Geometry: final body of the model. Coordinates: model frame, mm. A direction names the side the tool comes from. Round coordinates to 2 decimals unless told otherwise and drop trailing zeros. Loops run counter-clockwise (first coordinate to the right, second up) from the corner with the lowest first, then second, coordinate; pieces in that order, holes last. Notation, with made-up numbers: M 18.5,10 L 28.5,10 A28 cw 28.5,32 Z; hole C 81.5,60.25 d9. An arc over 180 degrees is marked long. Return JSON: item names as keys, results as strings.
from build123d import *

# Parameters (mm, degrees)
BOSS_EXTRUDE1_DEPTH = 15
CUT_EXTRUDE1_DEPTH  = 15
FILLET1_R           = 1


with BuildPart() as part:
    # Sketch1 → Boss-Extrude1 (new body)
    with BuildSketch(Plane.XY):
        Polygon((-6.3, 15.8), (1.3, 15.8), (1.3, 13.8), (1.3, 8.2), (-1.3, 8.2), (-1.3, 14), (-6.3, 14), align=None)
    extrude(amount=BOSS_EXTRUDE1_DEPTH)

    # Sketch3 → Cut-Extrude1 (cut)
    with BuildSketch(Plane(origin=(1.3, 0, 0), x_dir=(0, 0, -1), z_dir=(1, 0, 0))):
        Polygon((-15, 9.3), (-15.890506456, 6.842306326), (2.099726504, 7.064407967), (0, 10.3), align=None)
    extrude(amount=-CUT_EXTRUDE1_DEPTH, mode=Mode.SUBTRACT)

    # Fillet1
    fillet1_edges = [part.edges().sort_by_distance(p)[0] for p in [
        (0, 10.3, 0),
        (0, 9.3, 15),
    ]]
    fillet(fillet1_edges, radius=FILLET1_R)


solid = part.part
Q1. Reachability of faces 1 (the flat face through (-2, 15, 0)), 2 (the flat face through (-1.3, 12, 7)) from +Z, -Z, +X, -X, +Y, -Y: full face, straight path, thin tool, end or side. Return the list, or none.
Determined:
{"face 1": "-Z, +X, -X, +Y, -Y", "face 2": "+Z, -Z, -X, -Y"}
Q2. Section query C-C (y = 13.25). Output: boundary loops of the cut face in (x, z).
Determined:
{"outline": "M -1.3,0 L 1.3,0 L 1.3,15 L -1.3,15 Z"}
Q3. Section query B-B (z = 9). Output: boundary loops of the cut face in (x, y).
Determined:
{"outline": "M -6.3,14 L -1.3,14 L -1.3,9.7 L 1.3,9.7 L 1.3,15.8 L -6.3,15.8 Z"}
Q4. Pin query (flat end, axial travel): pin 1 (2 mm diameter, centred on x = -1.5, z = 3, fed in from -Y); pin 2 (1.5 mm diameter, centred on x = -4, z = 6.5, fed in from -Y); pin 3 (2.5 mm diameter, centred on y = 11, z = 8.5, fed in from -X). Return the tip coordinate at first contact, or that it passes through.
Determined:
{"pin 1": "stops at y = 10.03", "pin 2": "stops at y = 14", "pin 3": "stops at x = -1.3"}
Q5. Section query D-D (x = -3.5). Output: boundary loops of the cut face in (y, z), plus the area to 3 significant figures.
Determined:
{"outline": "M 14,0 L 15.8,0 L 15.8,15 L 14,15 Z", "area": "27.0 mm^2"}
Q6. Section query A-A (x = -1). Output: boundary loops of the cut face in (y, z).
Determined:
{"outline": "M 9.37,13.93 L 10.24,0.93 A1 ccw 11.24,0 L 15.8,0 L 15.8,15 L 10.37,15 A1 ccw Z"}
Q7. Material intervals for L1, parallel to X at y = 12.75, z = 10.25; L2, parallel to Y at x = -5.5, z = 4.25; L3, parallel to Y at x = 0.5, z = 2, sorted ascending.
Determined:
{"L1": "x = -1.3 to 1.3", "L2": "y = 14 to 15.8", "L3": "y = 10.17 to 15.8"}
